For this review, take the finished solid that the model builds, in its own axes (mm). A direction names the side the tool comes from. Round coordinates to 2 decimals unless told otherwise and drop trailing zeros. Loops run counter-clockwise (first coordinate to the right, second up) from the corner with the lowest first, then second, coordinate; pieces in that order, holes last. Notation, with made-up numbers: (9.5, 64.25) -> (52.5, 64.25) arc R20 ccw to (52.5, 79.25) -> close; hole circle Ø3 at (87, 81.5). An arc over 180 degrees is marked (long way). One line per question, with ' | ' between items. Start each with the question number.
1. Draft analysis for pull direction Y (two halves, no side actions). For faces 1 (the face through (101, 0, 0)), 2 (the face through (99, 0, 3)), state which applies: pulls with the +Y half, pulls with the -Y half, needs draft (parallel to the pull), parting line crosses it, or undercut.
2. For pin 1 Ø12 at (x, z) = (80.5, 72) entering from -Y; pin 2 Ø12 at (x, z) = (91, 142.5) entering from -Y; pin 3 Ø6 at (x, z) = (87.5, 169) entering from -Y, all flat-tipped, find the tip position at first contact; note any pin that passes through.
3. Consider section C-C (y = 25). Write out the cut boundary in (x, z).
4. Wall thickness on line 1 along Z through (x, y) = (99, -4); line 2 along Y through (x, z) = (62.5, 70); line 3 along Y through (x, z) = (60, 13): over which ranges is each line inside the solid? List them lowest first.
5. For faces 3 (the face through (99, 0, 2)), 4 (the face through (101, 0, 242)), list the 3-axis set-ups (+Z, -Z, +X, -X, +Y, -Y) from which the entire face can be reached by the end or side of a thin tool; tool diameter is ignored.
6. Consider section D-D (x = 89.5). Write out the cut boundary in (y, z).
7. Consider section B-B (z = 111.5). Write out the cut boundary in (x, y), and give its area (3 significant figures).
8. Consider section A-A (x = 69). Write out the cut boundary in (y, z), and give its area (3 significant figures).
```python
from build123d import *

# Parameters (mm, degrees)
EXTRUDE_1_DEPTH = 242
EXTRUDE_3_DEPTH = 1


with BuildPart() as part:
    # 草图1 → 凸台-拉伸1 (new body)
    with BuildSketch(Plane.XY):
        with BuildLine():
            Line((50, 52), (50, 50))
            ThreePointArc((50, 50), (62.940952255, 48.296291314), (75, 43.301270189))
            ThreePointArc((75, 43.301270189), (93.301270189, 25), (100, 0))
            ThreePointArc((100, 0), (93.301270189, -25), (75, -43.301270189))
            ThreePointArc((75, -43.301270189), (62.940952255, -48.296291314), (50, -50))
            Line((50, -50), (50, -52))
            ThreePointArc((50, -52), (63.458590345, -50.228142967), (76, -45.033320997))
            ThreePointArc((76, -45.033320997), (95.033320997, -26), (102, 0))
            ThreePointArc((102, 0), (95.033320997, 26), (76, 45.033320997))
            ThreePointArc((76, 45.033320997), (63.458590345, 50.228142967), (50, 52))
        make_face()
    extrude(amount=EXTRUDE_1_DEPTH)

    # 草图4 → 凸台-拉伸3 (add)
    with BuildSketch(Plane(origin=(0, 0, 2), x_dir=(-1, 0, 0), z_dir=(0, 0, -1))):
        with BuildLine():
            Line((-50, 50), (-50, 48))
            ThreePointArc((-50, 48), (-98, 0), (-50, -48))
            Line((-50, -48), (-50, -50))
            ThreePointArc((-50, -50), (-100, 0), (-50, 50))
        make_face()
    extrude(amount=-EXTRUDE_3_DEPTH)


solid = part.part
```
Answer block:
1) face 1: needs draft | face 2: undercut
2) pin 1: stops at y = -45.87 | pin 2: stops at y = -38.46 | pin 3: stops at y = -38.91
3) outline: (90.98, 2) -> (93.3, 2) -> (93.3, 0) -> (95.6, 0) -> (95.6, 242) -> (93.3, 242) -> (93.3, 3) -> (90.98, 3) -> close
4) line 1: z = 2 to 3 | line 2: y = -50.48 to -48.41, 48.41 to 50.48 | line 3: y = -51.03 to -48.99, 48.99 to 51.03
5) face 3: -Z, -X | face 4: +Z, +X, -X, +Y, -Y
6) outline: (-33.82, 0) -> (-30.66, 0) -> (-30.66, 2) -> (-27.27, 2) -> (-27.27, 3) -> (-30.66, 3) -> (-30.66, 242) -> (-33.82, 242) -> close; (27.27, 2) -> (30.66, 2) -> (30.66, 0) -> (33.82, 0) -> (33.82, 242) -> (30.66, 242) -> (30.66, 3) -> (27.27, 3) -> close
7) outline: (50, -52) arc R52 ccw to (50, 52) -> (50, 50) arc R50 cw to (50, -50) -> close | area: 320 mm2
8) outline: (-48.4, 0) -> (-46.25, 0) -> (-46.25, 2) -> (-44.08, 2) -> (-44.08, 3) -> (-46.25, 3) -> (-46.25, 242) -> (-48.4, 242) -> close; (44.08, 2) -> (46.25, 2) -> (46.25, 0) -> (48.4, 0) -> (48.4, 242) -> (46.25, 242) -> (46.25, 3) -> (44.08, 3) -> close | area: 1,050 mm2
